Source: CAD feature listing. Evaluate the final solid. Frame: model axes, mm. A direction names the side the tool comes from. Round coordinates to 2 decimals unless told otherwise and drop trailing zeros. Order: outer loops, then holes, each group sorted by start corner. A loop starts at its lowest first (then second) coordinate and runs counter-clockwise, first axis right, second up. Notation, with made-up numbers: M 23,14 L 28,14 A11 ccw 28,24 Z; hole C 87.5,24 d10. An arc over 180 degrees is marked long. Answer in a Markdown table with one row per item. Add a question column.
```python
from build123d import *

# Parameters (mm, degrees)
SOFT_CONTACT_AND_WRAP_START     = -1
SOFT_CONTACT_AND_WRAP_PROFILE_W = 22
SOFT_CONTACT_AND_WRAP_PROFILE_H = 7
SOFT_CONTACT_AND_WRAP_DEPTH     = 6
SLIP_POCKET_START               = -0.1
FIXED_BAR_SLIP_POCKET_PROFILE_W = 24
FIXED_BAR_SLIP_POCKET_PROFILE_H = 5.2
SLIP_POCKET_DEPTH               = 4.2
PAD_CAPTURE_M2_START            = -50
PAD_CAPTURE_M2_PROFILE_R        = 1.1
PAD_CAPTURE_M2_DEPTH            = 129.038452061


with BuildPart() as part:
    # Soft_contact_and_wrap_profile → Soft_contact_and_wrap (new body)
    with BuildSketch(Plane.XY.offset(SOFT_CONTACT_AND_WRAP_START)):
        with Locations((65, -13.5)):
            Rectangle(SOFT_CONTACT_AND_WRAP_PROFILE_W, SOFT_CONTACT_AND_WRAP_PROFILE_H)
    extrude(amount=SOFT_CONTACT_AND_WRAP_DEPTH)

    # Fixed_bar_slip_pocket_profile → Slip_pocket (cut)
    with BuildSketch(Plane.XY.offset(SLIP_POCKET_START)):
        with Locations((65, -13.5)):
            Rectangle(FIXED_BAR_SLIP_POCKET_PROFILE_W, FIXED_BAR_SLIP_POCKET_PROFILE_H)
    extrude(amount=SLIP_POCKET_DEPTH, mode=Mode.SUBTRACT)

    # Pad_capture_M2_profile → Pad_capture_M2 (cut, through all)
    with BuildSketch(Plane.XY.offset(PAD_CAPTURE_M2_START)):
        with Locations(Location((57, -13.5, 0), (0, 0, 180))):
            Circle(PAD_CAPTURE_M2_PROFILE_R)
        with Locations(Location((73, -13.5, 0), (0, 0, 180))):
            Circle(PAD_CAPTURE_M2_PROFILE_R)
    extrude(amount=PAD_CAPTURE_M2_DEPTH, mode=Mode.SUBTRACT)


solid = part.part
```
(1) Cut plane D-D (x = 63.75). Return loops of the section in (y, z).
(2) Pin query (flat end, axial travel): pin 1 (2 mm diameter, centred on x = 73, y = -13.5, fed in from +Z). Return the tip coordinate at first contact, or that it passes through.
(3) Cut plane C-C (x = 73). Return loops of the section in (y, z).
(4) Line query: line 1 (Z direction, x = 61.25, y = -15.75); line 2 (Y direction, x = 73, z = 4.45); line 3 (Y direction, x = 58, z = 3.7). Output: solid intervals per line, ascending. Write a range as from..to.
(5) Access query for faces 1 (the face through (76, -13.5, 4.6)), 2 (the face through (65, -10.9, 2)). Directions: +Z, -Z, +X, -X, +Y, -Y. A direction counts if a zero-diameter tool reaches every point of the face in a straight line with its end or side. Return the directions, or none.
(6) Draft query along Z for faces 3 (the face through (65, -13, -1)), 4 (the face through (57.87, -12.83, -0.56)), 5 (the face through (65, -13, -0.1)). Return one class per face: +Z half, -Z half, draft (parallel to the pull), parting line (faces both ways), or undercut.
(7) Cut plane A-A (y = -15.75). Return loops of the section in (x, z), and give its area (3 significant figures).
(8) Cut plane B-B (z = 3.6). Return loops of the section in (x, y), and give its area (3 significant figures).
Answer list:
| question | item | result |
|---|---|---|
| 1 | outline | M -17,-1 L -10,-1 L -10,5 L -17,5 Z; hole M -16.1,-0.1 L -10.9,-0.1 L -10.9,4.1 L -16.1,4.1 Z |
| 2 | pin 1 | through |
| 3 | outline | M -17,-1 L -14.6,-1 L -14.6,-0.1 L -16.1,-0.1 L -16.1,4.1 L -14.6,4.1 L -14.6,5 L -17,5 Z; M -12.4,-1 L -10,-1 L -10,5 L -12.4,5 L -12.4,4.1 L -10.9,4.1 L -10.9,-0.1 L -12.4,-0.1 Z |
| 4 | line 1 | -1..-0.1, 4.1..5 |
| 4 | line 2 | -17..-14.6, -12.4..-10 |
| 4 | line 3 | -17..-16.1, -10.9..-10 |
| 5 | face 1 | +Z, -Z, +X, +Y, -Y |
| 5 | face 2 | +X, -X |
| 6 | face 3 | -Z half |
| 6 | face 4 | draft |
| 6 | face 5 | undercut |
| 7 | outline | M 54,-1 L 76,-1 L 76,-0.1 L 54,-0.1 Z; M 54,4.1 L 76,4.1 L 76,5 L 54,5 Z |
| 7 | area | 39.6 mm² |
| 8 | outline | M 54,-17 L 76,-17 L 76,-16.1 L 54,-16.1 Z; M 54,-10.9 L 76,-10.9 L 76,-10 L 54,-10 Z |
| 8 | area | 39.6 mm² |
